Autodesk Inventor part; units mm, degrees
ref_plane "YZ Plane" through (0, 0, 0) normal (1, 0, 0) x (0, 1, 0)
ref_plane "XZ Plane" through (0, 0, 0) normal (0, 1, 0) x (-1, 0, 0)
ref_plane "XY Plane" through (0, 0, 0) normal (0, 0, 1) x (1, 0, 0)
sketch "Sketch1" plane through (0, 0, 0) normal (0, 0, 1) x (1, 0, 0)
  line L0 (0, 28) -> (2.75, 28)
  line L1 (2.75, 28) -> (2.75, 25)
  line L2 (2.75, 25) -> (1.5, 25)
  line L3 (1.5, 25) -> (1.5, 0)
  line L4 (1.5, 0) -> (0, 0)
  line L5 (0, 0) -> (0, 28)
  dimension "d0" = 2.75
  dimension "d1" = 3
  dimension "d2" = 25
  dimension "d3" = 1.5
revolve "Revolution1" add sketch "Sketch1" angle 360 about axis through (0, 0, 0) along (0, 1, 0)
thread "Thread1"
sketch "Sketch3" plane through (0, 28, 0) normal (0, 1, 0) x (1, 0, 0)
  line L0 (1.25, -0.7217) -> (0, -1.4434)
  line L1 (0, -1.4434) -> (-1.25, -0.7217)
  line L2 (-1.25, -0.7217) -> (-1.25, 0.7217)
  line L3 (-1.25, 0.7217) -> (0, 1.4434)
  line L4 (0, 1.4434) -> (1.25, 0.7217)
  line L5 (1.25, 0.7217) -> (1.25, -0.7217)
  point P0 (0, 0)
  point P1 (0, 0)
  dimension "d13" = 2.5
extrude "Extrusion2" cut sketch "Sketch3" against normal blind 1.5
chamfer "Chamfer2" distance 0.1 angle 45 16 edges at (0.625, 28, 1.0825) (1.25, 28, 0) (1.25, 26.5, 0) (0.625, 28, -1.0825) (0.625, 26.5, -1.0825) (-0.625, 28, -1.0825) (-0.625, 26.5, -1.0825) (-1.25, 26.5, 0) (-1.25, 28, 0) (-0.625, 26.5, 1.0825) (-0.625, 28, 1.0825) (0.625, 26.5, 1.0825) (-2.75, 28, 0) (-2.75, 25, 0) (-1.5, 25, 0) (-1.5, 0, 0)
properties part number "M3 X 25"
Here's how the part is built. I have some questions about the finished solid (model axes, mm). A direction names the side the tool comes from. Round coordinates to 2 decimals unless told otherwise and drop trailing zeros. Write each loop counter-clockwise with the first axis right and the second up, starting at its lowest first coordinate (ties: lowest second). Pieces come first, ordered by that corner, then holes.
Q1. Will these pins go through, and if not, where does the flat tip stop? P1, Ø1.2, axis at x = 0.5, z = 0.5, coming from the +Y side; P2, Ø1, axis at x = 0.5, z = -2, coming from the -Y side; P3, Ø1.5, axis at y = 14.5, z = 0, coming from the -X side.
Q2. If we mould it in two halves opening along Z, with no side actions, what happens to faces 4 (the flat face through (-0.63, 27.26, -1.08)), 5 (the cylindrical face through (-0.596, 26.48, -2.685)), 6 (the flat face through (-1.25, 27, 0)), 7 (the flat face through (0, 0, 0))? For each: +Z half, -Z half, draft (parallel to the pull), parting line (faces both ways), or undercut.
Q3. If we section it at B-B on y = 3.5: Write out the boundary of the cut face in (x, z), plus the area to 3 significant figures.
Q4. Which directions (+Z, -Z, +X, -X, +Y, -Y) give clear straight access to the entire face, cutting with the end or side of a thin tool? Please do faces 1 (the flat face through (1.25, 27, 0)), 2 (the cylindrical face through (-1.5, 12.33, 0.07)), 3 (the flat face through (1.1, 28, 1.1)).
Q5. If we section it at A-A on z = 0: Write out the boundary of the cut face in (x, y).
Q6. Please list where these lines run through material, in increasing order: probe 1 along Y at (x, z) = (2.25, 1.3); probe 2 along X at (y, z) = (25.25, -2.45); probe 3 along Y at (x, z) = (0.3, -0.05).
Answer below:
1. P1: stops at y = 27.93
1. P2: stops at y = 24.96
1. P3: stops at x = -1.5
2. face 4: undercut
2. face 5: parting line
2. face 6: undercut
2. face 7: draft
3. outline: circle Ø3 at (0, 0)
3. area: 7.07 mm2
4. face 1: +Y
4. face 2: -Y
4. face 3: +Z, -Z, +X, -X, +Y
5. outline: (-2.75, 25.1) - (-2.65, 25) - (-1.6, 25) - (-1.5, 24.9) - (-1.5, 0.1) - (-1.4, 0) - (1.4, 0) - (1.5, 0.1) - (1.5, 24.9) - (1.6, 25) - (2.65, 25) - (2.75, 25.1) - (2.75, 27.9) - (2.65, 28) - (1.35, 28) - (1.25, 27.9) - (1.25, 26.6) - (1.15, 26.5) - (-1.15, 26.5) - (-1.25, 26.6) - (-1.25, 27.9) - (-1.35, 28) - (-2.65, 28) - (-2.75, 27.9) - close
6. probe 1: y = 25 to 28
6. probe 2: x = -1.25 to 1.25
6. probe 3: y = 0 to 26.5
